```python
from build123d import *

# Parameters (mm, degrees)
BOSS_EXTRUDE1_DEPTH = 63.5
BOSS_EXTRUDE2_DEPTH = 12.7


with BuildPart() as part:
    # Sketch1 → Boss-Extrude1 (new body, symmetric)
    with BuildSketch(Plane(origin=(0, 0, 0), x_dir=(1, 0, 0), z_dir=(0, 1, 0))):
        with BuildLine():
            Line((104.032447095, 113.531493902), (102.959947641, 112.36106613))
            ThreePointArc((102.959947641, 112.36106613), (0, 152.4), (-102.959947641, 112.36106613))
            Line((-102.959947641, 112.36106613), (-104.032447095, 113.531493902))
            ThreePointArc((-104.032447095, 113.531493902), (0, 153.9875), (104.032447095, 113.531493902))
        make_face()
    extrude(amount=BOSS_EXTRUDE1_DEPTH, both=True)

    # Sketch2 → Boss-Extrude2 (add, symmetric)
    with BuildSketch(Plane(origin=(0, 0, 0), x_dir=(1, 0, 0), z_dir=(0, 1, 0))):
        with BuildLine():
            Line((73.025, 179.3875), (-73.025, 179.3875))
            ThreePointArc((-73.025, 179.3875), (-75.27006403, 178.45756403), (-76.2, 176.2125))
            Line((-76.2, 176.2125), (-76.2, 135.64534928))
            ThreePointArc((-76.2, 135.64534928), (-76.620744225, 134.065887306), (-77.771464646, 132.905039193))
            ThreePointArc((-77.771464646, 132.905039193), (-90.09671873, 124.878867028), (-101.6, 115.713396615))
            Line((-101.6, 115.713396615), (-102.64742268, 116.90631823))
            ThreePointArc((-102.64742268, 116.90631823), (-91.025550882, 126.166278029), (-78.573232323, 134.275194237))
            ThreePointArc((-78.573232323, 134.275194237), (-77.997872113, 134.855618293), (-77.7875, 135.64534928))
            Line((-77.7875, 135.64534928), (-77.7875, 176.2125))
            ThreePointArc((-77.7875, 176.2125), (-76.392596045, 179.580096045), (-73.025, 180.975))
            Line((-73.025, 180.975), (73.025, 180.975))
            ThreePointArc((73.025, 180.975), (76.392596045, 179.580096045), (77.7875, 176.2125))
            Line((77.7875, 176.2125), (77.7875, 135.64534928))
            ThreePointArc((77.7875, 135.64534928), (77.997872113, 134.855618293), (78.573232323, 134.275194237))
            ThreePointArc((78.573232323, 134.275194237), (91.025550882, 126.166278029), (102.64742268, 116.90631823))
            Line((102.64742268, 116.90631823), (101.6, 115.713396615))
            ThreePointArc((101.6, 115.713396615), (90.09671873, 124.878867028), (77.771464646, 132.905039193))
            ThreePointArc((77.771464646, 132.905039193), (76.620744225, 134.065887306), (76.2, 135.64534928))
            Line((76.2, 135.64534928), (76.2, 176.2125))
            ThreePointArc((76.2, 176.2125), (75.27006403, 178.45756403), (73.025, 179.3875))
        make_face()
    extrude(amount=BOSS_EXTRUDE2_DEPTH, both=True)


solid = part.part
```
Work out the finished part from the listing and answer in its coordinate system (mm). A direction names the side the tool comes from. Round coordinates to 2 decimals unless told otherwise and drop trailing zeros. Order: outer loops, then holes, each group sorted by start corner. A loop starts at its lowest first (then second) coordinate and runs counter-clockwise, first axis right, second up.
Q1. The mould has two halves that part along Z. Classify faces 1 (the cylindrical face through (-91.194, 0.178, -126.044)), 2 (the flat face through (1, 0, -179.388)), 3 (the flat face through (-76.2, 0, -156)), 4 (the flat face through (0, 63.5, -153)): pulls with the +Z half, pulls with the -Z half, needs draft (parallel to the pull), parting line crosses it, or undercut.
Solution:
face 1: pulls with the -Z half
face 2: undercut
face 3: undercut
face 4: needs draft
Q2. Given pin 1 Ø12.5 at (y, z) = (-6, -151) entering from -X; pin 2 Ø7.5 at (y, z) = (-4, -163) entering from +X; pin 3 Ø5 at (y, z) = (-24, -145) entering from +X, each flat-ended and moving along its own axis, determine where each tip first touches the part or whether it passes through.
Solution:
pin 1: stops at x = -77.79
pin 2: stops at x = 77.79
pin 3: stops at x = 58.36
Q3. A tool of negligible diameter and unlimited length cuts with its end or side. For faces 5 (the flat face through (0, -63.5, -153)), 6 (the flat face through (-77.788, 0, -156)), 7 (the flat face through (77.788, 0, -156)), 8 (the flat face through (76.2, 0, -156)), from which of +Z, -Z, +X, -X, +Y, -Y can it reach the whole face along a straight path? Write none if from no direction.
Solution:
face 5: +Z, -Z, +X, -X, -Y
face 6: -Z, -X, +Y, -Y
face 7: -Z, +X, +Y, -Y
face 8: +Y, -Y
Q4. A cutting plane is placed at C-C, the plane x = -29. Determine the outline of the cut face in (y, z) (1 decimal).
Solution:
outline: (-63.5, -151.2) - (63.5, -151.2) - (63.5, -149.6) - (-63.5, -149.6) - close; (-12.7, -181) - (12.7, -181) - (12.7, -179.4) - (-12.7, -179.4) - close
Q5. Find the intervals of material crossed by line 1 along Z through (x, y) = (-1, 2) (1 decimal); line 2 along X through (y, z) = (-3, -166); line 3 along X through (y, z) = (14, -139), in increasing order.
Solution:
line 1: z = -181 to -179.4, -154 to -152.4
line 2: x = -77.79 to -76.2, 76.2 to 77.79
line 3: x = -66.27 to -62.49, 62.49 to 66.27
Q6. A cutting plane is placed at A-A, the plane z = -162. Determine the outline of the cut face in (x, y), then the cut area to 3 significant figures.
Solution:
outline: (-77.79, -12.7) - (-76.2, -12.7) - (-76.2, 12.7) - (-77.79, 12.7) - close; (76.2, -12.7) - (77.79, -12.7) - (77.79, 12.7) - (76.2, 12.7) - close
area: 80.6 mm2
